Part model, mm, in its own coordinate system. Face numbers are marked on the shaded views. Give positions to 0.01 mm unless a question says otherwise; leave off trailing zeros. Write each loop counter-clockwise with the first axis right and the second up, starting at its lowest first coordinate (ties: lowest second). Pieces come first, ordered by that corner, then holes. Notation, with made-up numbers: M 16,66.25 L 28,66.25 A17 cw 28,93.25 Z; hole C 6.25,83 d11. An arc over 180 degrees is marked long. Use CSV: the item, a comma, the result in double quotes. Start each with the question number.
Item 1: Cut at A-A (y = 0). List the corners of the cut face in (x, z), then the cut area to 3 significant figures.
Item 2: Cut at D-D (y = 16.5). List the corners of the cut face in (x, z).
Item 3: Mould opens along X. For the marked faces 1, 2, 3 and 4 say: released by +X, released by -X, zero draft, split by the parting line, or undercut.
Item 4: Cut at B-B (x = -7.5). List the corners of the cut face in (y, z).
Item 5: Cut at C-C (z = 3.5). Count the separate pieces of the cut face and the enclosed holes in it, then the cut area to 3 significant figures.
Item 6: Pin check, flat tips, straight feed: pin 1 (1.7 mm diameter, centred on y = -10.5, z = 3, fed in from +X); pin 2 (3 mm diameter, centred on y = -12, z = 6, fed in from +X); pin 3 (0.5 mm diameter, centred on x = -32.5, z = 5.5, fed in from -Y); pin 4 (12 mm diameter, centred on x = -2, y = -9.5, fed in from -Z). Stop position of each tip, or through.
Item 7: Drill centre lines: line 1 (Y direction, x = -0.5, z = 8.5); line 2 (X direction, y = 1, z = 8.5); line 3 (Y direction, x = -35, z = 3.75). Where is each one in solid material? Low to high. Write a range as [from, to].
from build123d import *

# Parameters (mm, degrees)
F0_W     = 0.6460093453
F0_H     = 5.5586001861
F0_R     = 5
F0_W_2   = 0.6280364187
F0_H_2   = 5.4039517833
F1_DEPTH = 10


with BuildPart() as f1:
    # F0 (on Top) → F1 (new body)
    with BuildSketch(Plane.XY):
        with BuildLine():
            ThreePointArc((0, 21), (21, 0), (0, -21))
            Line((0, -21), (0, -30))
            ThreePointArc((0, -30), (6.5894949497, -29.2673633303), (12.8571428571, -27.1052370872))
            Line((12.8571428571, -27.1052370872), (41.4285714286, -13.5526185436))
            ThreePointArc((41.4285714286, -13.5526185436), (50, 0), (41.4285714286, 13.5526185436))
            Line((41.4285714286, 13.5526185436), (12.8571428571, 27.1052370872))
            ThreePointArc((12.8571428571, 27.1052370872), (6.5894949497, 29.2673633303), (0, 30))
            Line((0, 30), (0, 21))
        make_face()
        with BuildLine():
            add(Edge.make_bspline(
                [(21.3959532578, -8.5758308066), (23.4787555162, -8.5758308066), (23.4787555162, -10.1951122353)],
                knots=[0, 0, 0, 1, 1, 1], degree=2))
            add(Edge.make_bspline(
                [(23.4787555162, -10.1951122353), (23.4787555162, -11.0394257676), (22.9027001019, -11.4938221715)],
                knots=[0, 0, 0, 1, 1, 1], degree=2))
            add(Edge.make_bspline(
                [(22.9027001019, -11.4938221715), (22.3266446875, -11.9482185755), (21.2548288057, -11.9482185755)],
                knots=[0, 0, 0, 1, 1, 1], degree=2))
            Line((21.2548288057, -11.9482185755), (20.6003033297, -11.9482185755))
            Line((20.6003033297, -11.9482185755), (20.6003033297, -14.1344309927))
            Line((20.6003033297, -14.1344309927), (19.9542939844, -14.1344309927))
            Line((19.9542939844, -14.1344309927), (19.9542939844, -8.5758308066))
            Line((19.9542939844, -8.5758308066), (21.3959532578, -8.5758308066))
        make_face(mode=Mode.SUBTRACT)
        with Locations((24.9648203285, -11.3551308997)):
            Rectangle(F0_W, F0_H, mode=Mode.SUBTRACT)
        Polygon((29.9108673971, -14.1344309927), (26.8122124017, -14.1344309927), (26.8122124017, -8.5758308066), (27.458221747, -8.5758308066), (27.458221747, -13.5492511526), (29.9108673971, -13.5492511526), align=None, mode=Mode.SUBTRACT)
        Polygon((35.0168960644, -14.1344309927), (34.347771507, -14.1344309927), (33.6555317378, -12.3667255713), (31.427955257, -12.3667255713), (30.7442316184, -14.1344309927), (30.0897061424, -14.1344309927), (32.2868678705, -8.5527155947), (32.8306836471, -8.5527155947), align=None, mode=Mode.SUBTRACT)
        with BuildLine():
            Line((37.5875509545, -11.8229097947), (36.4269239951, -11.8229097947))
            Line((36.4269239951, -11.8229097947), (36.4269239951, -14.1344309927))
            Line((36.4269239951, -14.1344309927), (35.7809146498, -14.1344309927))
            Line((35.7809146498, -14.1344309927), (35.7809146498, -8.5758308066))
            Line((35.7809146498, -8.5758308066), (37.3053020503, -8.5758308066))
            add(Edge.make_bspline(
                [(37.3053020503, -8.5758308066), (38.328454328, -8.5758308066), (38.8169152548, -8.9675728202)],
                knots=[0, 0, 0, 1, 1, 1], degree=2))
            add(Edge.make_bspline(
                [(38.8169152548, -8.9675728202), (39.3053761816, -9.3593148337), (39.3053761816, -10.1464486312)],
                knots=[0, 0, 0, 1, 1, 1], degree=2))
            add(Edge.make_bspline(
                [(39.3053761816, -10.1464486312), (39.3053761816, -11.2486792655), (38.1873298759, -11.6367715088)],
                knots=[0, 0, 0, 1, 1, 1], degree=2))
            Line((38.1873298759, -11.6367715088), (39.6971181952, -14.1344309927))
            Line((39.6971181952, -14.1344309927), (38.9330996097, -14.1344309927))
            Line((38.9330996097, -14.1344309927), (37.5875509545, -11.8229097947))
        make_face(mode=Mode.SUBTRACT)
        with Locations((35, 0)):
            Circle(F0_R, mode=Mode.SUBTRACT)
        with BuildLine():
            Line((0, -30), (0, -21))
            ThreePointArc((0, -21), (-21, 0), (0, 21))
            Line((0, 21), (0, 30))
            ThreePointArc((0, 30), (-6.5894949497, 29.2673633303), (-12.8571428571, 27.1052370872))
            Line((-12.8571428571, 27.1052370872), (-41.4285714286, 13.5526185436))
            ThreePointArc((-41.4285714286, 13.5526185436), (-50, 0), (-41.4285714286, -13.5526185436))
            Line((-41.4285714286, -13.5526185436), (-12.8571428571, -27.1052370872))
            ThreePointArc((-12.8571428571, -27.1052370872), (-6.5894949497, -29.2673633303), (0, -30))
        make_face()
        with BuildLine():
            add(Edge.make_bspline(
                [(-38.4772362224, -6.8385926591), (-36.452380575, -6.8385926591), (-36.452380575, -8.4128233056)],
                knots=[0, 0, 0, 1, 1, 1], degree=2))
            add(Edge.make_bspline(
                [(-36.452380575, -8.4128233056), (-36.452380575, -9.2336467981), (-37.0124092836, -9.6754012282)],
                knots=[0, 0, 0, 1, 1, 1], degree=2))
            add(Edge.make_bspline(
                [(-37.0124092836, -9.6754012282), (-37.5724379921, -10.1171556583), (-38.6144343854, -10.1171556583)],
                knots=[0, 0, 0, 1, 1, 1], degree=2))
            Line((-38.6144343854, -10.1171556583), (-39.2507500036, -10.1171556583))
            Line((-39.2507500036, -10.1171556583), (-39.2507500036, -12.2425444424))
            Line((-39.2507500036, -12.2425444424), (-39.8787864223, -12.2425444424))
            Line((-39.8787864223, -12.2425444424), (-39.8787864223, -6.8385926591))
            Line((-39.8787864223, -6.8385926591), (-38.4772362224, -6.8385926591))
        make_face(mode=Mode.SUBTRACT)
        with Locations((-35.0076602635, -9.5405685508)):
            Rectangle(F0_W_2, F0_H_2, mode=Mode.SUBTRACT)
        Polygon((-30.1992194723, -12.2425444424), (-33.2116653449, -12.2425444424), (-33.2116653449, -6.8385926591), (-32.5836289263, -6.8385926591), (-32.5836289263, -11.673645163), (-30.1992194723, -11.673645163), align=None, mode=Mode.SUBTRACT)
        Polygon((-25.2352480049, -12.2425444424), (-25.8857565365, -12.2425444424), (-26.558737181, -10.5240191762), (-28.7243392198, -10.5240191762), (-29.3890406648, -12.2425444424), (-30.025356283, -12.2425444424), (-27.8893228138, -6.8161205462), (-27.360636789, -6.8161205462), align=None, mode=Mode.SUBTRACT)
        with Locations((-35, 0)):
            Circle(F0_R, mode=Mode.SUBTRACT)
        with BuildLine():
            Line((-22.7361125009, -9.9953331515), (-23.8644491175, -9.9953331515))
            Line((-23.8644491175, -9.9953331515), (-23.8644491175, -12.2425444424))
            Line((-23.8644491175, -12.2425444424), (-24.4924855361, -12.2425444424))
            Line((-24.4924855361, -12.2425444424), (-24.4924855361, -6.8385926591))
            Line((-24.4924855361, -6.8385926591), (-23.0105088269, -6.8385926591))
            add(Edge.make_bspline(
                [(-23.0105088269, -6.8385926591), (-22.015822145, -6.8385926591), (-21.5409509169, -7.2194358358)],
                knots=[0, 0, 0, 1, 1, 1], degree=2))
            add(Edge.make_bspline(
                [(-21.5409509169, -7.2194358358), (-21.0660796889, -7.6002790125), (-21.0660796889, -8.3655135942)],
                knots=[0, 0, 0, 1, 1, 1], degree=2))
            add(Edge.make_bspline(
                [(-21.0660796889, -8.3655135942), (-21.0660796889, -9.4370785571), (-22.153020308, -9.8143735054)],
                knots=[0, 0, 0, 1, 1, 1], degree=2))
            Line((-22.153020308, -9.8143735054), (-20.6852365122, -12.2425444424))
            Line((-20.6852365122, -12.2425444424), (-21.427998981, -12.2425444424))
            Line((-21.427998981, -12.2425444424), (-22.7361125009, -9.9953331515))
        make_face(mode=Mode.SUBTRACT)
    extrude(amount=F1_DEPTH)


solid = f1.part
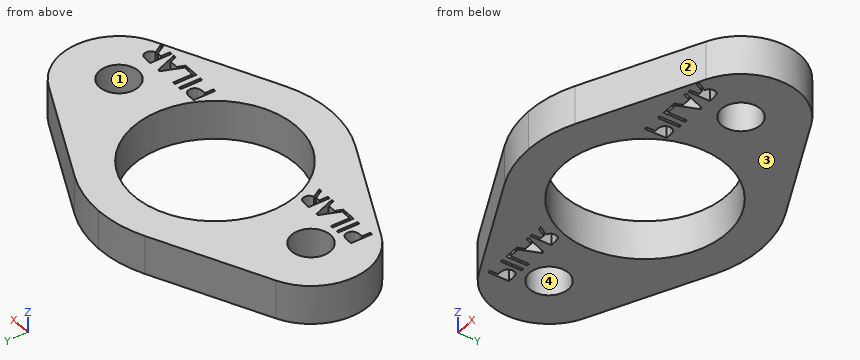
Worked answers:
1,outline,"M -50,0 L -40,0 L -40,10 L -50,10 Z; M -30,0 L -21,0 L -21,10 L -30,10 Z; M 21,0 L 30,0 L 30,10 L 21,10 Z; M 40,0 L 50,0 L 50,10 L 40,10 Z"
1,area,"380 mm^2"
2,outline,"M -35.21,0 L -12.99,0 L -12.99,10 L -35.21,10 Z; M 12.99,0 L 35.21,0 L 35.21,10 L 12.99,10 Z"
3,face 1,"undercut"
3,face 2,"released by +X"
3,face 3,"zero draft"
3,face 4,"undercut"
4,outline,"M -29.05,0 L -19.62,0 L -19.62,10 L -29.05,10 Z; M 19.62,0 L 29.05,0 L 29.05,10 L 19.62,10 Z"
5,separate pieces,"1"
5,enclosed holes,"13"
5,area,"2,520 mm^2"
6,pin 1,"stops at x = 46.48"
6,pin 2,"stops at x = 45.71"
6,pin 3,"stops at y = -17.91"
6,pin 4,"passes through"
7,line 1,"y = [-30, -20.99], [20.99, 30]"
7,line 2,"x = [-49.97, -39.9], [-30.1, -20.98], [20.98, 30.1], [39.9, 49.97]"
7,line 3,"y = [-16.6, -12.24], [-6.84, -5], [5, 16.6]"
